Here's the drawing with two shaded views (mm, measured from the low corner). I have some questions. A direction names the side the tool comes from. Give positions to 0.01 mm unless a question says otherwise; leave off trailing zeros. Loops run counter-clockwise (first coordinate to the right, second up) from the corner with the lowest first, then second, coordinate; pieces in that order, holes last. Notation, with made-up numbers: M -2.75,59 L 54.25,59 A14 cw 54.25,63 Z; hole C -33,39 d6. An arc over 180 degrees is marked long. Answer in a Markdown table with one row per item. Add a question column.
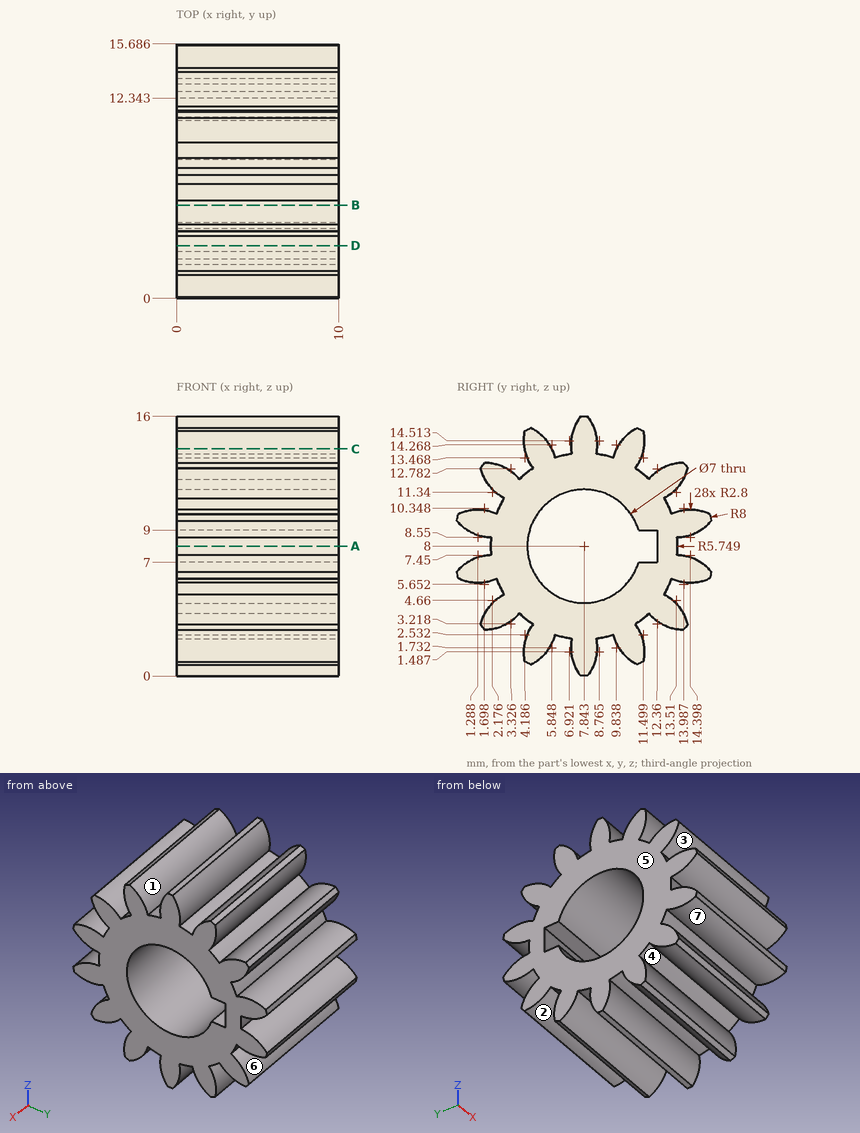
Item 1: Suppose I cut it at C-C (z = 14). Give the number of separate pieces and of enclosed holes in the cut face.
Item 2: Suppose I cut it at B-B (y = 5.75). List the corners of the cut face in (x, z) for me (1 decimal).
Item 3: Suppose I cut it at A-A (z = 8). List the corners of the cut face in (x, y) for me.
Item 4: For the marked faces 1, 2, 3 and 4, which set-ups out of +Z, -Z, +X, -X, +Y, -Y let a thin tool reach every point of the face, with its end or its side?
Item 5: I need wall thicknesses on L1, parallel to Y at x = 8.25, z = 8; L2, parallel to Y at x = 9.5, z = 3.5 (1 decimal); L3, parallel to Y at x = 5.75, z = 1.75 (1 decimal). Which ranges of each line are inside material? Lowest first, please.
Item 6: For P1, Ø4, axis at y = 7.84, z = 8, coming from the +X side; P2, Ø0.6, axis at x = 2.5, y = 11.5, coming from the +Z side; P3, Ø1, axis at x = 9, z = 2.5, coming from the -Y side; P4, Ø1.6, axis at x = 6.5, z = 8, coming from the -Y side (1 decimal), each with a flat end and sliding along its axis, tell me the tip position at first contact or that it passes through.
Item 7: Suppose I cut it at D-D (y = 3.25). List the corners of the cut face in (x, z) for me.
Item 8: If we mould it in two halves opening along Y, with no side actions, what happens to the marked faces 5, 6 and 7? For each: +Y half, -Y half, draft (parallel to the pull), parting line (faces both ways), or undercut.
Values found:
| question | item | result |
|---|---|---|
| 1 | separate pieces | 3 |
| 1 | enclosed holes | 0 |
| 2 | outline | M 0,1.8 L 10,1.8 L 10,5.2 L 0,5.2 Z; M 0,10.8 L 10,10.8 L 10,14.2 L 0,14.2 Z |
| 3 | outline | M 0,2.09 L 10,2.09 L 10,4.34 L 0,4.34 Z; M 0,12.34 L 10,12.34 L 10,13.59 L 0,13.59 Z |
| 4 | face 1 | +Z, +X, -X |
| 4 | face 2 | -Z, +X, -X |
| 4 | face 3 | +X, -X, -Y |
| 4 | face 4 | +X, -X |
| 5 | L1 | 2.09 to 4.34, 12.34 to 13.59 |
| 5 | L2 | 1.6 to 3.5, 4.3 to 11.4, 12.2 to 14.1 |
| 5 | L3 | 4.1 to 5.7, 7 to 8.6, 10 to 11.6 |
| 6 | P1 | through |
| 6 | P2 | z = 15.26 |
| 6 | P3 | y = 1.6 |
| 6 | P4 | y = 1 |
| 7 | outline | M 0,3.32 L 10,3.32 L 10,12.68 L 0,12.68 Z |
| 8 | face 5 | draft |
| 8 | face 6 | +Y half |
| 8 | face 7 | undercut |
